Source: CAD feature listing. Evaluate the final solid. Frame: model axes, mm. Round coordinates to 2 decimals unless told otherwise and drop trailing zeros. Write each loop counter-clockwise with the first axis right and the second up, starting at its lowest first coordinate (ties: lowest second). Pieces come first, ordered by that corner, then holes. Notation, with made-up numbers: M 35.25,-35.5 L 72.25,-35.5 A14 ccw 72.25,-24.5 Z; hole C 72,-18.75 d6. An arc over 180 degrees is marked long. Use a Markdown table: item, result.
Autodesk Inventor part; units mm, degrees
ref_plane "YZ Plane" through (0, 0, 0) normal (1, 0, 0) x (0, 1, 0)
ref_plane "XZ Plane" through (0, 0, 0) normal (0, 1, 0) x (-1, 0, 0)
ref_plane "XY Plane" through (0, 0, 0) normal (0, 0, 1) x (1, 0, 0)
sketch "Sketch1" plane through (0, 0, 0) normal (0, 0, 1) x (1, 0, 0)
  circle A0 centre (75, 150.5) radius 4.1881
  circle A1 centre (75, 61.5) radius 4.1881
  circle A2 centre (-75, 61.5) radius 4.1881
  circle A3 centre (-75, 150.5) radius 4.1881
  line L0 (-87.5, -2.5) -> (87.5, -2.5)
  line L1 (87.5, -2.5) -> (87.5, 115.5)
  line L2 (87.5, 115.5) -> (-87.5, 115.5)
  line L3 (-87.5, 115.5) -> (-87.5, -2.5)
  line L4 (-87.5, -2.5) -> (87.5, 115.5) construction
  line L5 (87.5, -2.5) -> (-87.5, 115.5) construction
  line L6 (47.5, 94) -> (-47.5, 94) construction
  line L7 (-47.5, 94) -> (-47.5, 19) construction
  line L8 (-47.5, 19) -> (47.5, 19) construction
  line L9 (47.5, 19) -> (47.5, 94) construction
  line L10 (47.5, 94) -> (-47.5, 19) construction
  line L11 (-47.5, 94) -> (47.5, 19) construction
  line L12 (75, 61.5) -> (-75, 61.5) construction
  line L13 (0, 61.5) -> (0, 56.5) construction
  point P0 (0, 0)
  dimension "d0" = 175
  dimension "d1" = 118
  dimension "d2" = 95
  dimension "d3" = 75
  dimension "d15" = 5
extrude "Extrusion1" add sketch "Sketch1" along normal blind 10 contours L3 L2 L1 L0
hole "Hole1" at (47.5, 94, 0) at (47.5, 19, 0) at (-47.5, 19, 0) at (-47.5, 94, 0) direction (0, 0, 1) diameter 8 depth 15
fillet "Fillet1" radius 4 4 edges at (87.5, 115.5, 5) (87.5, -2.5, 5) (-87.5, -2.5, 5) (-87.5, 115.5, 5)
fillet "Fillet2" radius 2 16 edges at (86.3284, 114.3284, 0) (0, 115.5, 0) (-86.3284, 114.3284, 0) (-87.5, 56.5, 0) (-86.3284, -1.3284, 0) (0, -2.5, 0) (86.3284, -1.3284, 0) (87.5, 56.5, 0) (86.3284, 114.3284, 10) (0, 115.5, 10) (-86.3284, 114.3284, 10) (-87.5, 56.5, 10) (-86.3284, -1.3284, 10) (0, -2.5, 10) (86.3284, -1.3284, 10) (87.5, 56.5, 10)
properties part number "CylinderSupport"
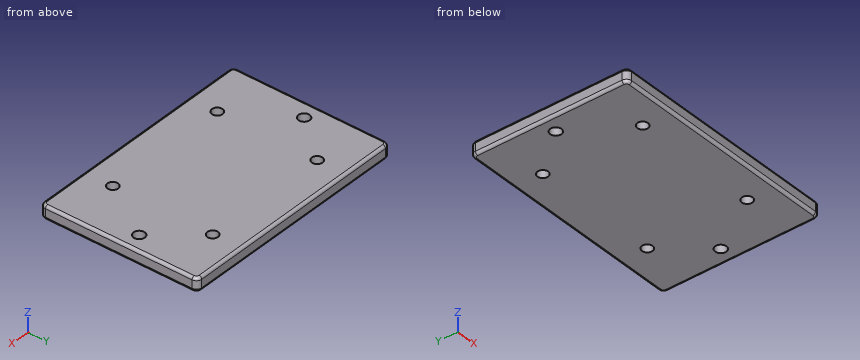
Q1. Section C-C on z = 4. Return loops of the section in (x, y), plus the area to 3 significant figures.
Results are:
| item | result |
|---|---|
| outline | M -87.5,1.5 A4 ccw -83.5,-2.5 L 83.5,-2.5 A4 ccw 87.5,1.5 L 87.5,111.5 A4 ccw 83.5,115.5 L -83.5,115.5 A4 ccw -87.5,111.5 Z; hole C -75,61.5 d8.38; hole C -47.5,19 d8; hole C -47.5,94 d8; hole C 47.5,19 d8; hole C 47.5,94 d8; hole C 75,61.5 d8.38 |
| area | 20,300 mm^2 |
Q2. Section B-B on y = 61.5. Return loops of the section in (x, z).
Results are:
| item | result |
|---|---|
| outline | M -87.5,2 A2 ccw -85.5,0 L -79.19,0 L -79.19,10 L -85.5,10 A2 ccw -87.5,8 Z; M -70.81,0 L 70.81,0 L 70.81,10 L -70.81,10 Z; M 79.19,0 L 85.5,0 A2 ccw 87.5,2 L 87.5,8 A2 ccw 85.5,10 L 79.19,10 Z |
Q3. Line query: L1, parallel to Y at x = 47.5, z = 5.5; L2, parallel to X at y = 94, z = 6.25; L3, parallel to X at y = 63, z = 9.5. Output: solid intervals per line, ascending.
Results are:
| item | result |
|---|---|
| L1 | -2.5 to 15, 23 to 90, 98 to 115.5 |
| L2 | -87.5 to -51.5, -43.5 to 43.5, 51.5 to 87.5 |
| L3 | -86.82 to -78.91, -71.09 to 71.09, 78.91 to 86.82 |
Q4. Section A-A on x = -75. Return loops of the section in (y, z), plus the area to 3 significant figures.
Results are:
| item | result |
|---|---|
| outline | M -2.5,2 A2 ccw -0.5,0 L 57.31,0 L 57.31,10 L -0.5,10 A2 ccw -2.5,8 Z; M 65.69,0 L 113.5,0 A2 ccw 115.5,2 L 115.5,8 A2 ccw 113.5,10 L 65.69,10 Z |
| area | 1,090 mm^2 |
